from build123d import *

# Parameters (mm, degrees)
BASE_FLANGE1_DEPTH         = 3.175
CUT_EXTRUDE1_DEPTH         = 3.175
CUT_EXTRUDE2_DEPTH         = 3.175
CUT_EXTRUDE3_DEPTH         = 291.545849439
CUT_EXTRUDE4_DEPTH         = 291.545849439
CUT_EXTRUDE5_DEPTH         = 291.545849439
CUT_EXTRUDE6_DEPTH         = 291.545849439
CUT_EXTRUDE7_DEPTH         = 291.545849439
CUT_EXTRUDE8_DEPTH         = 291.545849439
CUT_EXTRUDE9_DEPTH         = 291.545849439
CUT_EXTRUDE10_DEPTH        = 291.545849439
CUT_EXTRUDE11_DEPTH        = 291.545849439
F_4_2_4_2_DIAMETER_HOLE1_D = 4.2
F_5_2_5_2_DIAMETER_HOLE1_D = 5.2
F_3_5_3_5_DIAMETER_HOLE1_D = 3.5
F_3_2_3_2_DIAMETER_HOLE1_D = 3.2
F_5_0_5_DIAMETER_HOLE1_D   = 5
F_2_5_2_5_DIAMETER_HOLE1_D = 2.5


# Sheet-metal steps are written as plain solids
with BuildPart() as part:
    # Sketch11 → Base-Flange1 (new body)
    with BuildSketch(Plane(origin=(0, 32.675, 0), x_dir=(1, 0, 0), z_dir=(0, 1, 0))):
        with BuildLine():
            Line((222.001, 57.5), (222.001, 22))
            ThreePointArc((222.001, 22), (220.536533906, 18.464466094), (217.001, 17))
            Line((217.001, 17), (200.001, 17))
            ThreePointArc((200.001, 17), (196.465466094, 15.535533906), (195.001, 12))
            Line((195.001, 12), (195.001, -26.291796068))
            ThreePointArc((195.001, -26.291796068), (194.604567451, -27.487024677), (193.572428571, -28.208425763))
            ThreePointArc((193.572428571, -28.208425763), (190.001, -33), (193.572428571, -37.791574237))
            ThreePointArc((193.572428571, -37.791574237), (194.604567451, -38.512975323), (195.001, -39.708203932))
            Line((195.001, -39.708203932), (195.001, -43))
            ThreePointArc((195.001, -43), (200.858864376, -57.142135624), (215.001, -63))
            Line((215.001, -63), (255.001, -63))
            ThreePointArc((255.001, -63), (269.143135624, -57.142135624), (275.001, -43))
            Line((275.001, -43), (275.001, -39.708203932))
            ThreePointArc((275.001, -39.708203932), (275.397432549, -38.512975323), (276.429571429, -37.791574237))
            ThreePointArc((276.429571429, -37.791574237), (280.001, -33), (276.429571429, -28.208425763))
            ThreePointArc((276.429571429, -28.208425763), (275.397432549, -27.487024677), (275.001, -26.291796068))
            Line((275.001, -26.291796068), (275.001, 12))
            ThreePointArc((275.001, 12), (273.536533906, 15.535533906), (270.001, 17))
            Line((270.001, 17), (253.001, 17))
            ThreePointArc((253.001, 17), (249.465466094, 18.464466094), (248.001, 22))
            Line((248.001, 22), (248.001, 57.5))
            ThreePointArc((248.001, 57.5), (249.465466094, 61.035533906), (253.001, 62.5))
            Line((253.001, 62.5), (256.501, 62.5))
            ThreePointArc((256.501, 62.5), (260.036533906, 63.964466094), (261.501, 67.5))
            Line((261.501, 67.5), (261.501, 72.5))
            ThreePointArc((261.501, 72.5), (260.036533906, 76.035533906), (256.501, 77.5))
            Line((256.501, 77.5), (213.501, 77.5))
            ThreePointArc((213.501, 77.5), (209.965466094, 76.035533906), (208.501, 72.5))
            Line((208.501, 72.5), (208.501, 67.5))
            ThreePointArc((208.501, 67.5), (209.965466094, 63.964466094), (213.501, 62.5))
            Line((213.501, 62.5), (217.001, 62.5))
            ThreePointArc((217.001, 62.5), (220.536533906, 61.035533906), (222.001, 57.5))
        make_face()
    extrude(amount=-BASE_FLANGE1_DEPTH)

    # Sketch16 → Cut-Extrude1 (cut)
    with BuildSketch(Plane.XZ.offset(-29.5)):
        with BuildLine():
            Line((222.001, -35), (222.001, -35.230121613))
            Line((222.001, -35.230121613), (222.006298403, -35.230121613))
            ThreePointArc((222.006298403, -35.230121613), (222.002324776, -35.1150913), (222.001, -35))
        make_face()
    extrude(amount=-CUT_EXTRUDE1_DEPTH, mode=Mode.SUBTRACT)

    # Sketch17 → Cut-Extrude2 (cut)
    with BuildSketch(Plane.XZ.offset(-29.5)):
        with BuildLine():
            Line((248.001, -35.230121613), (248.001, -35))
            ThreePointArc((248.001, -35), (247.999675224, -35.1150913), (247.995701597, -35.230121613))
            Line((247.995701597, -35.230121613), (248.001, -35.230121613))
        make_face()
    extrude(amount=-CUT_EXTRUDE2_DEPTH, mode=Mode.SUBTRACT)

    # Sketch18 → Cut-Extrude3 (cut, through all)
    with BuildSketch(Plane(origin=(0, 32.675, 0), x_dir=(-1, 0, 0), z_dir=(0, 1, 0))):
        with BuildLine():
            Line((-250.001, 13), (-220.001, 13))
            ThreePointArc((-220.001, 13), (-200.001, 33), (-220.001, 53))
            Line((-220.001, 53), (-250.001, 53))
            ThreePointArc((-250.001, 53), (-270.001, 33), (-250.001, 13))
        make_face()
    extrude(amount=-CUT_EXTRUDE3_DEPTH, mode=Mode.SUBTRACT)

    # Sketch19 → Cut-Extrude4 (cut, through all)
    with BuildSketch(Plane(origin=(0, 32.675, 0), x_dir=(-1, 0, 0), z_dir=(0, 1, 0))):
        with BuildLine():
            Line((-225.001, -33), (-225.001, -23))
            ThreePointArc((-225.001, -23), (-227.001, -21), (-229.001, -23))
            Line((-229.001, -23), (-229.001, -33))
            ThreePointArc((-229.001, -33), (-227.001, -35), (-225.001, -33))
        make_face()
    extrude(amount=-CUT_EXTRUDE4_DEPTH, mode=Mode.SUBTRACT)

    # Sketch20 → Cut-Extrude5 (cut, through all)
    with BuildSketch(Plane(origin=(0, 32.675, 0), x_dir=(-1, 0, 0), z_dir=(0, 1, 0))):
        with BuildLine():
            Line((-241.001, -33), (-241.001, -23))
            ThreePointArc((-241.001, -23), (-243.001, -21), (-245.001, -23))
            Line((-245.001, -23), (-245.001, -33))
            ThreePointArc((-245.001, -33), (-243.001, -35), (-241.001, -33))
        make_face()
    extrude(amount=-CUT_EXTRUDE5_DEPTH, mode=Mode.SUBTRACT)

    # Sketch21 → Cut-Extrude6 (cut, through all)
    with BuildSketch(Plane(origin=(0, 32.675, 0), x_dir=(-1, 0, 0), z_dir=(0, 1, 0))):
        with BuildLine():
            Line((-225.501, -51.5), (-225.501, -48.5))
            ThreePointArc((-225.501, -48.5), (-228.001, -46), (-230.501, -48.5))
            Line((-230.501, -48.5), (-230.501, -51.5))
            ThreePointArc((-230.501, -51.5), (-228.001, -54), (-225.501, -51.5))
        make_face()
    extrude(amount=-CUT_EXTRUDE6_DEPTH, mode=Mode.SUBTRACT)

    # Sketch22 → Cut-Extrude7 (cut, through all)
    with BuildSketch(Plane(origin=(0, 32.675, 0), x_dir=(-1, 0, 0), z_dir=(0, 1, 0))):
        with BuildLine():
            Line((-239.501, -51.5), (-239.501, -48.5))
            ThreePointArc((-239.501, -48.5), (-242.001, -46), (-244.501, -48.5))
            Line((-244.501, -48.5), (-244.501, -51.5))
            ThreePointArc((-244.501, -51.5), (-242.001, -54), (-239.501, -51.5))
        make_face()
    extrude(amount=-CUT_EXTRUDE7_DEPTH, mode=Mode.SUBTRACT)

    # Sketch23 → Cut-Extrude8 (cut, through all)
    with BuildSketch(Plane(origin=(0, 32.675, 0), x_dir=(-1, 0, 0), z_dir=(0, 1, 0))):
        with BuildLine():
            Line((-211.501, -71.5), (-211.501, -68.5))
            ThreePointArc((-211.501, -68.5), (-214.001, -66), (-216.501, -68.5))
            Line((-216.501, -68.5), (-216.501, -71.5))
            ThreePointArc((-216.501, -71.5), (-214.001, -74), (-211.501, -71.5))
        make_face()
    extrude(amount=-CUT_EXTRUDE8_DEPTH, mode=Mode.SUBTRACT)

    # Sketch24 → Cut-Extrude9 (cut, through all)
    with BuildSketch(Plane(origin=(0, 32.675, 0), x_dir=(-1, 0, 0), z_dir=(0, 1, 0))):
        with BuildLine():
            Line((-225.501, -71.5), (-225.501, -68.5))
            ThreePointArc((-225.501, -68.5), (-228.001, -66), (-230.501, -68.5))
            Line((-230.501, -68.5), (-230.501, -71.5))
            ThreePointArc((-230.501, -71.5), (-228.001, -74), (-225.501, -71.5))
        make_face()
    extrude(amount=-CUT_EXTRUDE9_DEPTH, mode=Mode.SUBTRACT)

    # Sketch25 → Cut-Extrude10 (cut, through all)
    with BuildSketch(Plane(origin=(0, 32.675, 0), x_dir=(-1, 0, 0), z_dir=(0, 1, 0))):
        with BuildLine():
            Line((-239.501, -71.5), (-239.501, -68.5))
            ThreePointArc((-239.501, -68.5), (-242.001, -66), (-244.501, -68.5))
            Line((-244.501, -68.5), (-244.501, -71.5))
            ThreePointArc((-244.501, -71.5), (-242.001, -74), (-239.501, -71.5))
        make_face()
    extrude(amount=-CUT_EXTRUDE10_DEPTH, mode=Mode.SUBTRACT)

    # Sketch26 → Cut-Extrude11 (cut, through all)
    with BuildSketch(Plane.XZ.offset(-29.5)):
        with BuildLine():
            Line((253.501, -68.5), (253.501, -71.5))
            ThreePointArc((253.501, -71.5), (256.001, -74), (258.501, -71.5))
            Line((258.501, -71.5), (258.501, -68.5))
            ThreePointArc((258.501, -68.5), (256.001, -66), (253.501, -68.5))
        make_face()
    extrude(amount=-CUT_EXTRUDE11_DEPTH, mode=Mode.SUBTRACT)

    # Ø4.2 (4.2) Diameter Hole1 (through all)
    with Locations(Plane(origin=(0, 32.675, 0), x_dir=(1, 0, 0), z_dir=(0, 1, 0))):
        with Locations((215.001, -8), (215.001, -58), (255.001, -8), (235.001, -58), (255.001, -58), (235.001, -8)):
            Hole(F_4_2_4_2_DIAMETER_HOLE1_D / 2)

    # Ø5.2 (5.2) Diameter Hole1 (through all)
    with Locations(Plane(origin=(0, 32.675, 0), x_dir=(1, 0, 0), z_dir=(0, 1, 0))):
        with Locations((275.001, -33), (195.001, -33)):
            Hole(F_5_2_5_2_DIAMETER_HOLE1_D / 2)

    # Ø3.5 (3.5) Diameter Hole1 (through all)
    with Locations(Plane(origin=(0, 32.675, 0), x_dir=(1, 0, 0), z_dir=(0, 1, 0))):
        with Locations((202.001, -53), (268.001, -13), (202.001, -13), (268.001, -53)):
            Hole(F_3_5_3_5_DIAMETER_HOLE1_D / 2)

    # Ø3.2 (3.2) Diameter Hole1 (through all)
    with Locations(Plane(origin=(0, 32.675, 0), x_dir=(1, 0, 0), z_dir=(0, 1, 0))):
        with Locations((247.501, -58), (222.501, -58)):
            Hole(F_3_2_3_2_DIAMETER_HOLE1_D / 2)

    # Ø5.0 (5) Diameter Hole1 (through all)
    with Locations(Plane(origin=(0, 32.675, 0), x_dir=(1, 0, 0), z_dir=(0, 1, 0))):
        with Locations((242.001, 10), (228.001, 10), (270.001, 10), (256.001, 10), (214.001, 10), (200.001, 10)):
            Hole(F_5_0_5_DIAMETER_HOLE1_D / 2)

    # Ø2.5 (2.5) Diameter Hole1 (through all)
    with Locations(Plane(origin=(0, 32.675, 0), x_dir=(1, 0, 0), z_dir=(0, 1, 0))):
        with Locations((235.001, 23), (235.001, 33)):
            Hole(F_2_5_2_5_DIAMETER_HOLE1_D / 2)


solid = part.part
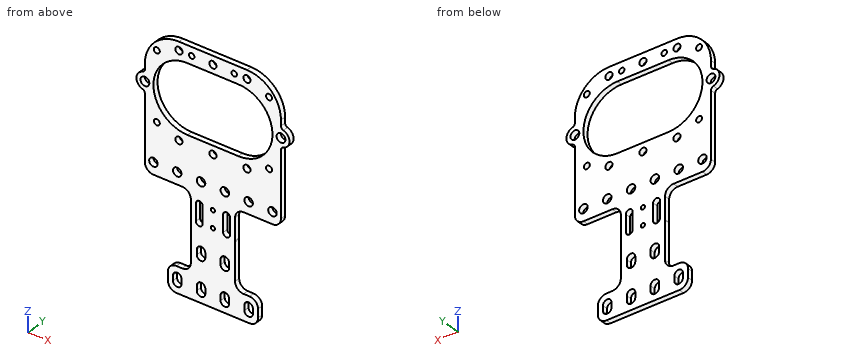
Can you work these out from the model? Positions are in its coordinate system, mm. Coordinates: 2 decimals unless noted, no trailing zeros. Write each loop counter-clockwise with the first axis right and the second up, starting at its lowest first coordinate (ties: lowest second). Pieces come first, ordered by that corner, then holes. Notation, with made-up numbers: (65, 55.25) - (79, 55.25) arc R13 ccw to (79, 65.25) - close; hole circle Ø9 at (55.5, 22.25). An arc over 180 degrees is marked (long way). Return JSON: item names as keys, results as strings. Group by question number.
Item 1: If we section it at B-B (z = 24.5): Write out the boundary of the cut face in (x, y) (3 decimals), then the cut area to 3 significant figures.
Item 2: If we section it at D-D (z = -39.5): Write out the boundary of the cut face in (x, y) (3 decimals), then the cut area to 4 significant figures.
Item 3: If we section it at C-C (y = 30.85): Count the separate pieces of the cut face and the enclosed holes in it, then the cut area to 3 significant figures.
Item 4: Please list where these lines run through material, in increasing order: probe 1 along X at (y, z) = (30.9, -51); probe 2 along Z at (x, y) = (238.5, 31.95); probe 3 along Z at (x, y) = (235.5, 30.9).
Item 5: I'm going to push flat-ended pins straight in: pin 1 Ø1.6 at (y, z) = (32, -47.5) entering from -X; pin 2 Ø1.6 at (y, z) = (31, -71) entering from -X; pin 3 Ø3 at (x, z) = (268.001, 53) entering from -Y; pin 4 Ø1 at (y, z) = (31, -27) entering from +X. Where does each tip first touch, or does it pass through?
Item 6: If we section it at A-A (x = 263): Write out the boundary of the cut face in (y, z) (3 decimals), then the cut area to 3 significant figures.
Return value:
{
 "1": {"outline": "(195.001, 29.5) - (201.897, 29.5) - (201.897, 32.675) - (195.001, 32.675) - close; (268.105, 29.5) - (275.001, 29.5) - (275.001, 32.675) - (268.105, 32.675) - close", "area": "43.8 mm^2"},
 "2": {"outline": "(222.001, 29.5) - (248.001, 29.5) - (248.001, 32.675) - (222.001, 32.675) - close", "area": "82.55 mm^2"},
 "3": {"separate pieces": "1", "enclosed holes": "31", "area": "5,200 mm^2"},
 "4": {"probe 1": "x = 222 to 225.5, 230.5 to 239.5, 244.5 to 248", "probe 2": "z = -77.5 to 13, 53 to 63", "probe 3": "z = -77.5 to -34.15, -31.85 to -24.15, -21.85 to 5.96, 10.04 to 13, 53 to 55.96, 60.04 to 63"},
 "5": {"pin 1": "stops at x = 222", "pin 2": "stops at x = 208.5", "pin 3": "passes through", "pin 4": "stops at x = 248"},
 "6": {"outline": "(29.5, -17) - (32.675, -17) - (32.675, 17.8) - (29.5, 17.8) - close; (29.5, 48.2) - (32.675, 48.2) - (32.675, 61.331) - (29.5, 61.331) - close", "area": "152 mm^2"}
}
